Verification items for the finished model (mm, model axes). Face numbers are marked on the shaded views. A direction names the side the tool comes from. Round coordinates to 2 decimals unless told otherwise and drop trailing zeros. Order: outer loops, then holes, each group sorted by start corner. A loop starts at its lowest first (then second) coordinate and runs counter-clockwise, first axis right, second up. Notation, with made-up numbers: (-24.5, -2.5) -> (14.5, -2.5) arc R16 cw to (14.5, 23.5) -> close; hole circle Ø10 at (73, 8.25). An arc over 180 degrees is marked (long way). Put each result on its own line as item: value.
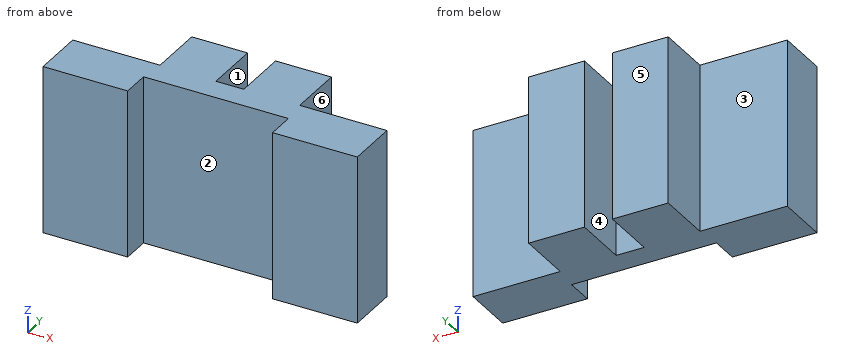
from build123d import *

# Parameters (mm, degrees)
SKETCH1_W           = 9
SKETCH1_H           = 4.8
BOSS_EXTRUDE1_DEPTH = 1.5
SKETCH2_W           = 4.15
SKETCH2_H           = 4.8
CUT_EXTRUDE1_DEPTH  = 0.8
SKETCH3_W           = 1.6
SKETCH3_H           = 4.8
BOSS_EXTRUDE2_DEPTH = 1.6


with BuildPart() as part:
    # Sketch1 → Boss-Extrude1 (new body)
    with BuildSketch(Plane(origin=(0, 0, 0), x_dir=(1, 0, 0), z_dir=(0, 1, 0))):
        Rectangle(SKETCH1_W, SKETCH1_H)
    extrude(amount=BOSS_EXTRUDE1_DEPTH)

    # Sketch2 → Cut-Extrude1 (cut)
    with BuildSketch(Plane(origin=(0, 0, 0), x_dir=(-1, 0, 0), z_dir=(0, -1, 0))):
        Rectangle(SKETCH2_W, SKETCH2_H)
    extrude(amount=-CUT_EXTRUDE1_DEPTH, mode=Mode.SUBTRACT)

    # Sketch3 → Boss-Extrude2 (add)
    with BuildSketch(Plane(origin=(0, 1.5, 0), x_dir=(1, 0, 0), z_dir=(0, 1, 0))):
        with Locations((1.2, 0)):
            Rectangle(SKETCH3_W, SKETCH3_H)
        with Locations((-1.2, 0)):
            Rectangle(SKETCH3_W, SKETCH3_H)
    extrude(amount=BOSS_EXTRUDE2_DEPTH)


solid = part.part
Item 1: Gauge pin test, flat ends, axial feed: pin 1 Ø2 at (x, z) = (-0.5, 0.5) entering from -Y; pin 2 Ø0.8 at (y, z) = (2.5, -0.5) entering from -X; pin 3 Ø1.2 at (x, z) = (-3, 0) entering from +Y; pin 4 Ø1.8 at (y, z) = (2, -1) entering from +X. Record the tip position at first contact, or that the pin passes through.
Check sheet entries:
pin 1: stops at y = 0.8
pin 2: stops at x = -2
pin 3: stops at y = 1.5
pin 4: stops at x = 4.5
Item 2: Section check C-C on y = 2.25. Record the boundary of the cut face in (x, z).
Check sheet entries:
outline: (-2, -2.4) -> (-0.4, -2.4) -> (-0.4, 2.4) -> (-2, 2.4) -> close; (0.4, -2.4) -> (2, -2.4) -> (2, 2.4) -> (0.4, 2.4) -> close
Item 3: Material ranges on L1, parallel to X at y = 2.55, z = -1.55; L2, parallel to X at y = 0.35, z = -0.55 (3 decimals); L3, parallel to Y at x = -1.75, z = 1.5, recorded low to high. Write a range as [from, to].
Check sheet entries:
L1: x = [-2, -0.4], [0.4, 2]
L2: x = [-4.5, -2.075], [2.075, 4.5]
L3: y = [0.8, 3.1]
Item 4: Section check B-B on z = -0.4. Record the boundary of the cut face in (x, y) (3 decimals).
Check sheet entries:
outline: (-4.5, 0) -> (-2.075, 0) -> (-2.075, 0.8) -> (2.075, 0.8) -> (2.075, 0) -> (4.5, 0) -> (4.5, 1.5) -> (2, 1.5) -> (2, 3.1) -> (0.4, 3.1) -> (0.4, 1.5) -> (-0.4, 1.5) -> (-0.4, 3.1) -> (-2, 3.1) -> (-2, 1.5) -> (-4.5, 1.5) -> close
Item 5: Section check A-A on y = 0.7. Record the boundary of the cut face in (x, z) (3 decimals), then the cut area to 3 significant figures.
Check sheet entries:
outline: (-4.5, -2.4) -> (-2.075, -2.4) -> (-2.075, 2.4) -> (-4.5, 2.4) -> close; (2.075, -2.4) -> (4.5, -2.4) -> (4.5, 2.4) -> (2.075, 2.4) -> close
area: 23.3 mm^2
Item 6: Section check D-D on x = -2.75. Record the boundary of the cut face in (y, z).
Check sheet entries:
outline: (0, -2.4) -> (1.5, -2.4) -> (1.5, 2.4) -> (0, 2.4) -> close
Item 7: Release check for a two-part mould opening along X. For the marked faces 4, 5 and 6 record: +X half, -X half, draft (parallel to the pull), parting line (faces both ways), or undercut.
Check sheet entries:
face 4: undercut
face 5: draft
face 6: +X half
Item 8: Tool access check on the marked faces 1, 2 and 3. Record the directions out of +Z, -Z, +X, -X, +Y, -Y that give a thin tool (end or side, any length) a straight path to the whole face; none if there is none.
Check sheet entries:
face 1: +Z, -Z, +Y
face 2: +Z, -Z, -Y
face 3: +Z, -Z, -X, +Y
